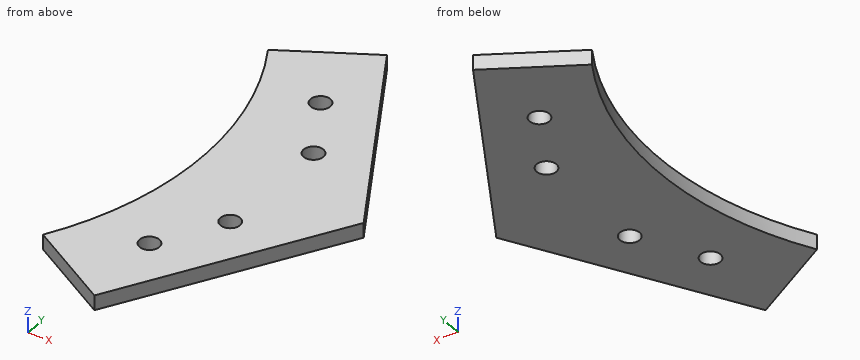
from build123d import *

# Parameters (mm, degrees)
SKETCH_1_R      = 2
EXTRUDE_1_DEPTH = 3


with BuildPart() as part:
    # 草图1 → 凸台-拉伸1 (new body)
    with BuildSketch(Plane.XY):
        with BuildLine():
            Line((30.874609077, -1.112961222), (5.874609077, 42.188308967))
            Line((5.874609077, 42.188308967), (-11.445898998, 32.188308967))
            ThreePointArc((-11.445898998, 32.188308967), (-2.522850544, -1.112961222), (-11.445898998, -34.414231411))
            Line((-11.445898998, -34.414231411), (5.874609077, -44.414231411))
            Line((5.874609077, -44.414231411), (30.874609077, -1.112961222))
        make_face()
        with Locations((4.714355039, -26.423850355)):
            Circle(SKETCH_1_R, mode=Mode.SUBTRACT)
        with Locations((12.214355039, -13.433469298)):
            Circle(SKETCH_1_R, mode=Mode.SUBTRACT)
        with Locations((12.214355039, 11.207546854)):
            Circle(SKETCH_1_R, mode=Mode.SUBTRACT)
        with Locations((4.714355039, 24.19792791)):
            Circle(SKETCH_1_R, mode=Mode.SUBTRACT)
    extrude(amount=EXTRUDE_1_DEPTH)


solid = part.part
Geometry: final body of the model. Coordinates: model frame, mm. Round coordinates to 2 decimals unless told otherwise and drop trailing zeros. Write each loop counter-clockwise with the first axis right and the second up, starting at its lowest first coordinate (ties: lowest second). Pieces come first, ordered by that corner, then holes. Notation, with made-up numbers: M 1,-23.5 L 6,-23.5 A30 ccw 6,8.5 Z; hole C -9.5,26.5 d11. An arc over 180 degrees is marked long. Write item = value, one per line.
Item 1: Section query A-A on y = -27.5. Return loops of the section in (x, z).
Findings:
outline = M -7.97,0 L 3.03,0 L 3.03,3 L -7.97,3 Z; M 6.4,0 L 15.64,0 L 15.64,3 L 6.4,3 Z
Item 2: Section query B-B on z = 1.55. Return loops of the section in (x, y), then the cut area to 3 significant figures.
Findings:
outline = M -11.45,-34.41 L 5.87,-44.41 L 30.87,-1.11 L 5.87,42.19 L -11.45,32.19 A66.6 cw Z; hole C 4.71,-26.42 d4; hole C 4.71,24.2 d4; hole C 12.21,-13.43 d4; hole C 12.21,11.21 d4
area = 1,960 mm^2
Item 3: Section query D-D on y = 0. Return loops of the section in (x, z), then the cut area to 3 significant figures.
Findings:
outline = M -2.53,0 L 30.23,0 L 30.23,3 L -2.53,3 Z
area = 98.3 mm^2
Item 4: Pin query (flat end, axial travel): P1, Ø1, axis at x = 22, z = 1, coming from the -Y side; P2, Ø1, axis at y = 25.5, z = 0.5, coming from the +X side. Return the tip coordinate at first contact, or that it passes through.
Findings:
P1 = -17.35
P2 = 15.8
Item 5: Section query C-C on x = 23. Return loops of the section in (y, z), then the cut area to 3 significant figures.
Findings:
outline = M -14.75,0 L 12.53,0 L 12.53,3 L -14.75,3 Z
area = 81.8 mm^2
Item 6: Material intervals for line 1 along Y through (x, z) = (4, 1.2); line 2 along Y through (x, z) = (3, 2.7); line 3 along X through (y, z) = (-14, 1.25), sorted ascending. Write a range as [from, to].
Findings:
line_1 = [-43.33, -28.29], [-24.56, 22.33], [26.07, 41.11]
line_2 = [-42.75, -27.45], [-25.39, 23.17], [25.23, 40.53]
line_3 = [-3.78, 10.3], [14.13, 23.43]
